```python
from build123d import *

# Parameters (mm, degrees)
F1_DEPTH = 444.5
F2_SIZE  = 76.19999
F3_SIZE  = 76.19999
F4_R     = 4.7625
F5_DEPTH = 25.4
F6_DEPTH = 25.4


# Not quite as in the source:
# - a fillet or chamfer is up to 0.001 mm smaller than in the source, because OpenCascade refuses the exact size


with BuildPart() as f1:
    # F0 (on Front) → F1 (new body, symmetric)
    with BuildSketch(Plane.XZ):
        with BuildLine():
            Line((34.6709999669, 34.4712352276), (-3.4290000331, 34.4712352276))
            Line((-3.4290000331, 34.4712352276), (-3.4290000331, -41.7287647724))
            Line((-3.4290000331, -41.7287647724), (34.6709999669, -41.7287647724))
            Line((34.6709999669, -41.7287647724), (34.6709999669, -41.1254357918))
            ThreePointArc((34.6709999669, -41.1254357918), (33.029223555, -36.864552005), (28.9528485827, -34.806949634))
            Line((28.9528485827, -34.806949634), (8.6391513512, -32.7755799108))
            ThreePointArc((8.6391513512, -32.7755799108), (4.5627763789, -30.7179775398), (2.9209999669, -26.457093753))
            Line((2.9209999669, -26.457093753), (2.9209999669, 19.1995642082))
            ThreePointArc((2.9209999669, 19.1995642082), (4.5627763789, 23.460447995), (8.6391513512, 25.518050366))
            Line((8.6391513512, 25.518050366), (28.9528485827, 27.5494200892))
            ThreePointArc((28.9528485827, 27.5494200892), (33.029223555, 29.6070224602), (34.6709999669, 33.867906247))
            Line((34.6709999669, 33.867906247), (34.6709999669, 34.4712352276))
        make_face()
    extrude(amount=F1_DEPTH, both=True)

    # F2 (size 76.2 in the source; OpenCascade refuses exactly that, so slightly less here)
    f2_edges = [f1.edges().sort_by_distance(p)[0] for p in [
        (15.621, -444.5, 34.471235),
    ]]
    chamfer(f2_edges, length=F2_SIZE)

    # F3 (size 76.2 in the source; OpenCascade refuses exactly that, so slightly less here)
    f3_edges = [f1.edges().sort_by_distance(p)[0] for p in [
        (15.621, 444.5, 34.471235),
    ]]
    chamfer(f3_edges, length=F3_SIZE)

    # F4 (on face) → F5 (cut)
    with BuildSketch(Plane(origin=(0, 0, -41.7287647724), x_dir=(1, 0, 0), z_dir=(0, 0, -1))):
        with Locations((21.9709999669, 425.45)):
            Circle(F4_R)
    extrude(amount=-F5_DEPTH, mode=Mode.SUBTRACT)

    # F4 (on face) → F6 (cut)
    with BuildSketch(Plane(origin=(0, 0, -41.7287647724), x_dir=(1, 0, 0), z_dir=(0, 0, -1))):
        with Locations((21.9709999669, 425.45)):
            Circle(F4_R)
        with Locations((21.9709999669, -425.45)):
            Circle(F4_R)
    extrude(amount=-F6_DEPTH, mode=Mode.SUBTRACT)


solid = f1.part
```
Here's how the part is built. I have some questions about the finished solid (model axes, mm). A direction names the side the tool comes from. Coordinates: 2 decimals unless noted, no trailing zeros. Order: outer loops, then holes, each group sorted by start corner. A loop starts at its lowest first (then second) coordinate and runs counter-clockwise, first axis right, second up. Notation, with made-up numbers: M 0.5,-16 L 47.5,-16 A20 cw 47.5,4 Z; hole C -26.75,14 d11. An arc over 180 degrees is marked long. Answer as a JSON object with one key per item and string values. Group by question number.
(1) For pin 1 (3 mm diameter, centred on y = -100.5, z = 20, fed in from +X); pin 2 (8 mm diameter, centred on x = 2.5, z = 24, fed in from +Y); pin 3 (23 mm diameter, centred on y = -162, z = -7.5, fed in from +X), each with a flat end and sliding along its axis, tell me the tip position at first contact or that it passes through.
(2) Suppose I cut it at A-A, the plane y = -255. Please give me the cut outline in (x, z).
(3) I need wall thicknesses on probe 1 along Z at (x, y) = (28, -183); probe 2 along Z at (x, y) = (8.5, 137.5); probe 3 along X at (y, z) = (425.45, -38). Which ranges of each line are inside material? Lowest first, please.
(4) Which directions (+Z, -Z, +X, -X, +Y, -Y) give clear straight access to the entire face, cutting with the end or side of a thin tool? Please do faces 4 (the face through (-3.429, -6, -3)), 5 (the face through (2.921, -6, -4)).
(5) If we mould it in two halves opening along Z, with no side actions, what happens to faces 1 (the face through (18.9, -6.1, -33.8)), 2 (the face through (15, -6, -41.729)), 3 (the face through (1.599, 403.756, -0.984))? For each: released by +Z, released by -Z, zero draft, split by the parting line, or undercut.
Values found:
{
 "1": {"pin 1": "stops at x = 3.35", "pin 2": "stops at y = 382.77", "pin 3": "stops at x = 2.92"},
 "2": {"outline": "M -3.43,-41.73 L 34.67,-41.73 L 34.67,-41.13 A6.35 ccw 28.95,-34.81 L 8.64,-32.78 A6.35 cw 2.92,-26.46 L 2.92,19.2 A6.35 cw 8.64,25.52 L 28.95,27.55 A6.35 ccw 34.67,33.87 L 34.67,34.47 L -3.43,34.47 Z"},
 "3": {"probe 1": "z = -41.73 to -34.71, 27.45 to 34.47", "probe 2": "z = -41.73 to -32.76, 25.5 to 34.47", "probe 3": "x = -3.43 to 17.21, 26.73 to 33.85"},
 "4": {"face 4": "+Z, -Z, -X, +Y, -Y", "face 5": "+X, +Y, -Y"},
 "5": {"face 1": "undercut", "face 2": "released by -Z", "face 3": "released by +Z"}
}
